Source: three-view drawing plus pictorial views. Frame: mm from the lowest corner of the part. A direction names the side the tool comes from. Coordinates: 2 decimals unless noted, no trailing zeros. Loops run counter-clockwise (first coordinate to the right, second up) from the corner with the lowest first, then second, coordinate; pieces in that order, holes last. Notation, with made-up numbers: (-5, 83.5) - (4, 83.5) arc R31 cw to (4, 112.5) - close; hole circle Ø4 at (46.25, -15.5). An arc over 180 degrees is marked (long way). Return JSON: item names as keys, results as strings.
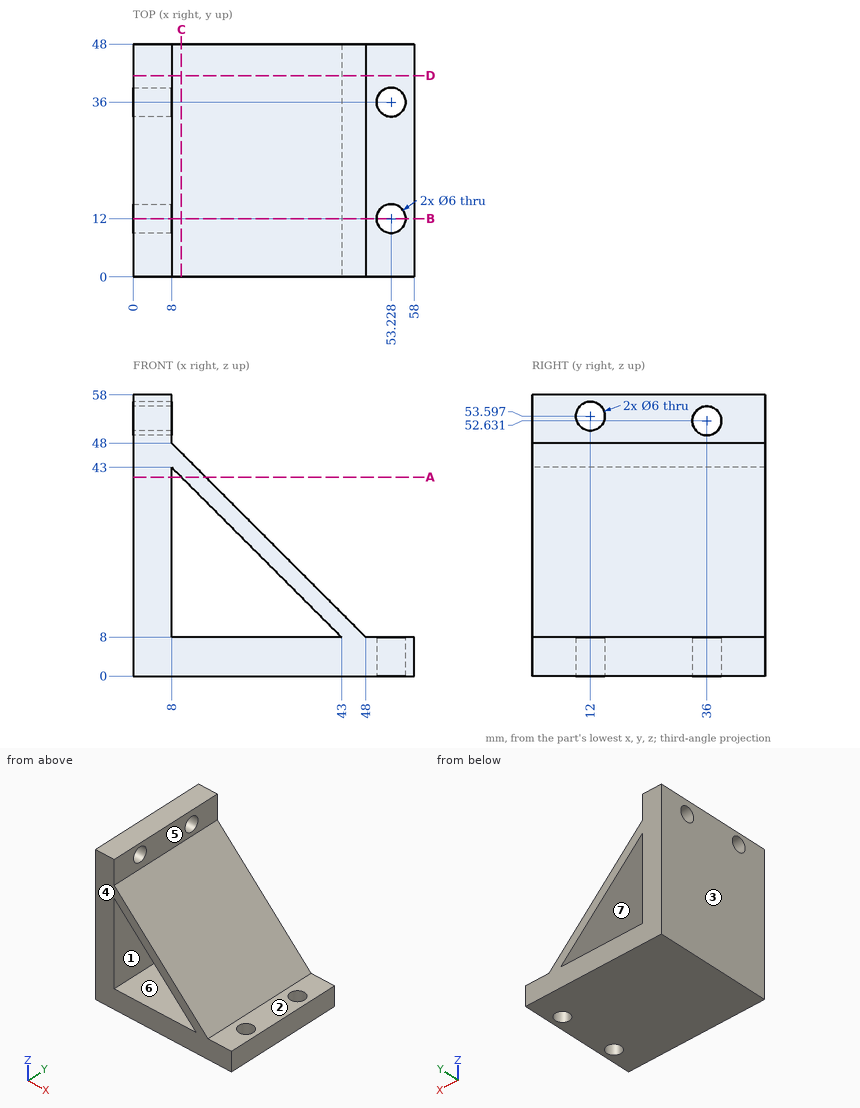
Item 1: Section query D-D, the plane y = 41.5. Return loops of the section in (x, z).
Worked out:
{"outline": "(0, 0) - (58, 0) - (58, 8) - (48, 8) - (8, 48) - (8, 58) - (0, 58) - close; hole (8, 8) - (43, 8) - (8, 43) - close"}
Item 2: Ray query, probe 1 along X at (y, z) = (12, 6); probe 2 along Z at (x, y) = (3.75, 12); probe 3 along Y at (x, z) = (53.5, 2.5). Return the intervals inside material, ascending. Write a range as from..to.
Worked out:
{"probe 1": "0..50.23, 56.23..58", "probe 2": "0..50.6, 56.6..58", "probe 3": "0..9.01, 14.99..33.01, 38.99..48"}
Item 3: Reachability of the marked faces 1, 2 and 3 from +Z, -Z, +X, -X, +Y, -Y: full face, straight path, thin tool, end or side. Return the list, or none.
Worked out:
{"face 1": "+Y, -Y", "face 2": "+Z, +X, +Y, -Y", "face 3": "+Z, -Z, -X, +Y, -Y"}
Item 4: Section query B-B, the plane y = 12. Return loops of the section in (x, z).
Worked out:
{"outline": "(0, 0) - (50.23, 0) - (50.23, 8) - (48, 8) - (8, 48) - (8, 50.6) - (0, 50.6) - close; (0, 56.6) - (8, 56.6) - (8, 58) - (0, 58) - close; (56.23, 0) - (58, 0) - (58, 8) - (56.23, 8) - close; hole (8, 8) - (43, 8) - (8, 43) - close"}
Item 5: First-contact query: pin 1 Ø1.5 at (x, y) = (8, 31) entering from -Z; pin 2 Ø2 at (y, z) = (23, 37.5) entering from +X; pin 3 Ø8 at (y, z) = (25, 53) entering from +X; pin 4 Ø5 at (y, z) = (20, 33.5) entering from +X. Flat tips, straight axial feed; report the tip coordinate or a pass-through.
Worked out:
{"pin 1": "z = 0", "pin 2": "x = 19.5", "pin 3": "x = 8", "pin 4": "x = 25"}
Item 6: Section query A-A, the plane z = 41. Return loops of the section in (x, y), and give its area (3 significant figures).
Worked out:
{"outline": "(0, 0) - (8, 0) - (8, 48) - (0, 48) - close; (10, 0) - (15, 0) - (15, 48) - (10, 48) - close", "area": "624 mm^2"}
Item 7: Mould query, pull axis X, two halves, no side actions, for the marked faces 4, 5, 6 and 7. Classes: +X half, -X half, draft (parallel to the pull), parting line (faces both ways), or undercut.
Worked out:
{"face 4": "draft", "face 5": "+X half", "face 6": "undercut", "face 7": "undercut"}
Item 8: Section query C-C, the plane x = 10. Return loops of the section in (y, z).
Worked out:
{"outline": "(0, 0) - (48, 0) - (48, 8) - (0, 8) - close; (0, 41) - (48, 41) - (48, 46) - (0, 46) - close"}
